Model file for the job. Use its own axes, mm. Face numbers are marked on the shaded views. A direction names the side the tool comes from. Coordinates: 2 decimals unless noted, no trailing zeros. Order: outer loops, then holes, each group sorted by start corner. A loop starts at its lowest first (then second) coordinate and runs counter-clockwise, first axis right, second up. Notation, with made-up numbers: M 4,42 L 53,42 A19 cw 53,77 Z; hole C -38.75,-39 d3. An arc over 180 degrees is marked long. Return JSON: item names as keys, results as strings.
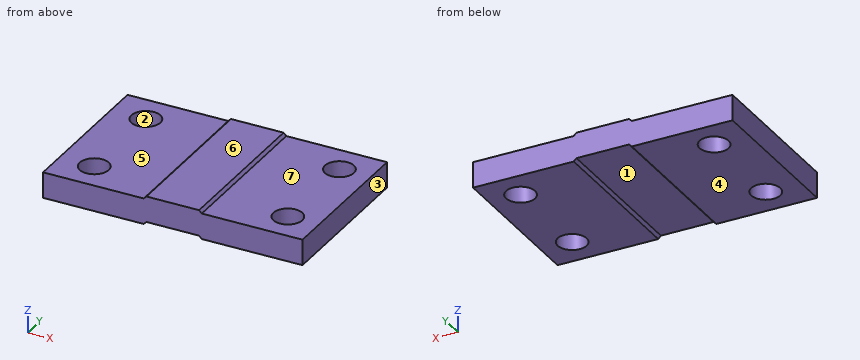
```python
from build123d import *

# Parameters (mm, degrees)
F1_DEPTH = 13.32
F4_DEPTH = 82.081
F7_DEPTH = 82.08
F9_D     = 15


with BuildPart() as f1:
    # F0 (on Top) → F1 (new body)
    with BuildSketch(Plane.XY):
        Polygon((-67.04, 0), (0, 0), (67.04, 0), (67.04, 82.08), (-67.04, 82.08), align=None)
    extrude(amount=F1_DEPTH)

    # F3 (on offset) → F4 (cut, through all)
    with BuildSketch(Plane.XZ):
        Polygon((-15, 0), (0, 0), (15, 0), (13.6, 1.4), (-13.6, 1.4), align=None)
    extrude(amount=-F4_DEPTH, mode=Mode.SUBTRACT)

    # F6 (on offset) → F7 (join)
    with BuildSketch(Plane.XZ):
        Polygon((-15, 13.32), (0, 13.32), (15, 13.32), (13.6, 14.72), (-13.6, 14.72), align=None)
    extrude(amount=-F7_DEPTH)

    # F9 (through all)
    with Locations(Plane(origin=(0, 0, 0), x_dir=(1, 0, 0), z_dir=(0, 0, -1))):
        with Locations((-49.04, -66.08), (-49.04, -16), (50.96, -16), (50.96, -66.08)):
            Hole(F9_D / 2)


solid = f1.part
```
Item 1: 3-axis set-ups, long thin cutter, end or side, ignore diameter. For the marked faces 5, 6 and 7: which of +Z, -Z, +X, -X, +Y, -Y reach the whole face in a straight line?
Check result:
{"face 5": "+Z, -X, +Y, -Y", "face 6": "+Z, +X, -X, +Y, -Y", "face 7": "+Z, +X, +Y, -Y"}
Item 2: Drop flat-ended pins along their axis: pin 1 Ø17 at (x, y) = (-49.04, 66.08) entering from +Z; pin 2 Ø10 at (x, y) = (5.5, 63.5) entering from -Z; pin 3 Ø9 at (x, y) = (50.96, 16) entering from +Z. Give the stop position or say it passes through.
Check result:
{"pin 1": "stops at z = 13.32", "pin 2": "stops at z = 1.4", "pin 3": "passes through"}
Item 3: Saw through at C-C (z = 4.25). Write the cut outline in (x, y), and give its area (3 significant figures).
Check result:
{"outline": "M -67.04,0 L 67.04,0 L 67.04,82.08 L -67.04,82.08 Z; hole C -49.04,16 d15; hole C -49.04,66.08 d15; hole C 50.96,16 d15; hole C 50.96,66.08 d15", "area": "10,300 mm2"}
Item 4: Pull direction X, two halves, no side cores. Call the marked faces 1, 2, 3 and 4: +X half, -X half, draft (parallel to the pull), parting line (faces both ways), or undercut.
Check result:
{"face 1": "undercut", "face 2": "undercut", "face 3": "+X half", "face 4": "draft"}
Item 5: Saw through at A-A (x = 50.96). Write the cut outline in (y, z), and give its area (3 significant figures).
Check result:
{"outline": "M 0,0 L 8.5,0 L 8.5,13.32 L 0,13.32 Z; M 23.5,0 L 58.58,0 L 58.58,13.32 L 23.5,13.32 Z; M 73.58,0 L 82.08,0 L 82.08,13.32 L 73.58,13.32 Z", "area": "694 mm2"}
Item 6: Saw through at B-B (y = 66.08). Write the cut outline in (x, z), and give its area (3 significant figures).
Check result:
{"outline": "M -67.04,0 L -56.54,0 L -56.54,13.32 L -67.04,13.32 Z; M -41.54,0 L -15,0 L -13.6,1.4 L 13.6,1.4 L 15,0 L 43.46,0 L 43.46,13.32 L 15,13.32 L 13.6,14.72 L -13.6,14.72 L -15,13.32 L -41.54,13.32 Z; M 58.46,0 L 67.04,0 L 67.04,13.32 L 58.46,13.32 Z", "area": "1,390 mm2"}
Item 7: Saw through at D-D (y = 48). Write the cut outline in (x, z).
Check result:
{"outline": "M -67.04,0 L -15,0 L -13.6,1.4 L 13.6,1.4 L 15,0 L 67.04,0 L 67.04,13.32 L 15,13.32 L 13.6,14.72 L -13.6,14.72 L -15,13.32 L -67.04,13.32 Z"}
Item 8: Wall check: line 1 (X direction, y = 66.08, z = 9.5); line 2 (Y direction, x = 50.96, z = 10.25); line 3 (X direction, y = 16.5, z = 7.5). Give the ranges that are in metal, low to high.
Check result:
{"line 1": "x = -67.04 to -56.54, -41.54 to 43.46, 58.46 to 67.04", "line 2": "y = 0 to 8.5, 23.5 to 58.58, 73.58 to 82.08", "line 3": "x = -67.04 to -56.52, -41.56 to 43.48, 58.44 to 67.04"}
